Could you check a few things on this model? Use its own coordinates, in mm. Face numbers are marked on the shaded views. A direction names the side the tool comes from. Give positions to 0.01 mm unless a question says otherwise; leave off trailing zeros. Loops run counter-clockwise (first coordinate to the right, second up) from the corner with the lowest first, then second, coordinate; pieces in that order, holes last. Notation, with made-up numbers: M 79.5,73.5 L 111.5,73.5 A13 ccw 111.5,86.5 Z; hole C 50.25,-39 d11. An arc over 180 degrees is marked long. Use a Markdown table: item, result. Add a question column.
1) Will these pins go through, and if not, where does the flat tip stop? pin 1 Ø12.5 at (y, z) = (-20, 16.5) entering from -X; pin 2 Ø7.5 at (y, z) = (-60.5, 13.5) entering from +X; pin 3 Ø1 at (x, z) = (-1, 86.5) entering from -Y.
2) If I drill on line 1 along Y through (x, z) = (-47.5, 110.5); line 2 along Y through (x, z) = (-110, 92.5); line 3 along Z through (x, y) = (98, -99), over which ranges is the centre line in solid material (lowest first)? Write a range as [from, to].
3) We'd pull the mould along X, two halves only. Please class the marked faces 4, 5, 6 and 7: +X half, -X half, draft (parallel to the pull), parting line (faces both ways), or undercut.
4) Which directions (+Z, -Z, +X, -X, +Y, -Y) give clear straight access to the entire face, cutting with the end or side of a thin tool? Please do the marked faces 1, 2 and 3.
5) Suppose I cut it at A-A on y = -31. List the corners of the cut face in (x, z) for me, and give its area (3 significant figures).
6) Suppose I cut it at C-C on z = 55. List the corners of the cut face in (x, y) for me.
7) Suppose I cut it at D-D on z = 114.5. List the corners of the cut face in (x, y) for me.
8) Suppose I cut it at B-B on x = -107.5. List the corners of the cut face in (y, z) for me, and give its area (3 significant figures).
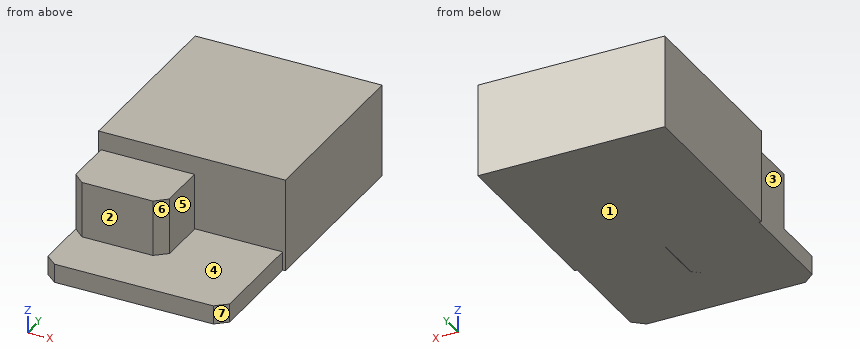
```python
from build123d import *

# Parameters (mm, degrees)
F0_W     = 254
F0_H     = 254
F2_DEPTH = 127
F3_DEPTH = 101.6
F5_DEPTH = 25.4


with BuildPart() as f2:
    # F0 (on Top) → F2 (new body)
    with BuildSketch(Plane.XY):
        with Locations((-4.570606, 150.885063)):
            Rectangle(F0_W, F0_H)
    extrude(amount=F2_DEPTH)

    # F1 (on face) → F3 (join)
    with BuildSketch(Plane.XY):
        Polygon((-1.268606, 23.885063), (-128.268606, 23.885063), (-128.268606, -42.154937), (-113.028606, -55.595354), (-16.508606, -55.595354), (-1.268606, -42.154937), align=None)
    extrude(amount=F3_DEPTH)

    # F4 (on Top) → F5 (join)
    with BuildSketch(Plane.XY):
        Polygon((103.190219, -128.514937), (118.749044, -115.44492), (118.749044, 23.885063), (-0.630956, 23.885063), (-0.630956, -42.154937), (-16.189781, -55.224955), (-112.709781, -55.224955), (-128.268606, -42.154937), (-128.268606, -115.44492), (-112.709781, -128.514937), align=None)
    extrude(amount=F5_DEPTH)


solid = f2.part
```
Answer block:
| question | item | result |
|---|---|---|
| 1 | pin 1 | stops at x = -128.27 |
| 1 | pin 2 | stops at x = 118.75 |
| 1 | pin 3 | stops at y = -42.36 |
| 2 | line 1 | y = [23.89, 277.89] |
| 2 | line 2 | y = [-55.6, 277.89] |
| 2 | line 3 | z = [0, 25.4] |
| 3 | face 4 | draft |
| 3 | face 5 | undercut |
| 3 | face 6 | undercut |
| 3 | face 7 | +X half |
| 4 | face 1 | -Z, +X, -X, +Y, -Y |
| 4 | face 2 | +Z, +X, -X, -Y |
| 4 | face 3 | +Z, -Z, -X, -Y |
| 5 | outline | M -128.27,0 L -1.27,0 L -1.27,101.6 L -128.27,101.6 Z; M -0.63,0 L 118.75,0 L 118.75,25.4 L -0.63,25.4 Z |
| 5 | area | 15,900 mm^2 |
| 6 | outline | M -131.57,23.89 L -128.27,23.89 L -128.27,-42.15 L -113.03,-55.6 L -16.51,-55.6 L -1.27,-42.15 L -1.27,23.89 L 122.43,23.89 L 122.43,277.89 L -131.57,277.89 Z |
| 7 | outline | M -131.57,23.89 L 122.43,23.89 L 122.43,277.89 L -131.57,277.89 Z |
| 8 | outline | M -128.51,0 L 277.89,0 L 277.89,127 L 23.89,127 L 23.89,101.6 L -55.6,101.6 L -55.6,25.4 L -128.51,25.4 Z |
| 8 | area | 42,200 mm^2 |
